Autodesk Inventor part; units mm, degrees
ref_plane "YZ Plane" through (0, 0, 0) normal (1, 0, 0) x (0, 1, 0)
ref_plane "XZ Plane" through (0, 0, 0) normal (0, 1, 0) x (-1, 0, 0)
ref_plane "XY Plane" through (0, 0, 0) normal (0, 0, 1) x (1, 0, 0)
sketch "Náčrt1" plane through (0, 0, 0) normal (0, 0, 1) x (1, 0, 0)
  line L0 (2.5, -1.4434) -> (0, -2.8868)
  line L1 (0, -2.8868) -> (-2.5, -1.4434)
  line L2 (-2.5, -1.4434) -> (-2.5, 1.4434)
  line L3 (-2.5, 1.4434) -> (0, 2.8868)
  line L4 (0, 2.8868) -> (2.5, 1.4434)
  line L5 (2.5, 1.4434) -> (2.5, -1.4434)
  circle A0 centre (0, 0) radius 1.5
  point P0 (2.5, 0)
  dimension "d1" = 3
  dimension "d16" = 5
extrude "Vysunutí1" add sketch "Náčrt1" along normal blind 20
thread "Závit1"
sketch "Náčrt2" plane through (0, 0, 20) normal (0, 0, 1) x (1, 0, 0)
  circle A0 centre (0, 0) radius 2.5
  dimension "d18" = 5
extrude "Vysunutí2" cut sketch "Náčrt2" against normal through all draft 45 keep common part
sketch "Náčrt3" plane through (0, 0, 0) normal (0, 0, -1) x (-1, 0, 0)
  circle A0 centre (0, 0) radius 2.5
  dimension "d17" = 5
extrude "Vysunutí3" cut sketch "Náčrt3" against normal through all draft 45 keep common part
chamfer "Zkosení1" distance 0.2 angle 45 1 edges at (-1.5, 0, 20)
chamfer "Zkosení2" distance 0.2 angle 45 1 edges at (-1.5, 0, 0)
properties part number "PillarBolt-M3x20" material "Ocel, vysokopevnostní, nízkolegovaná"
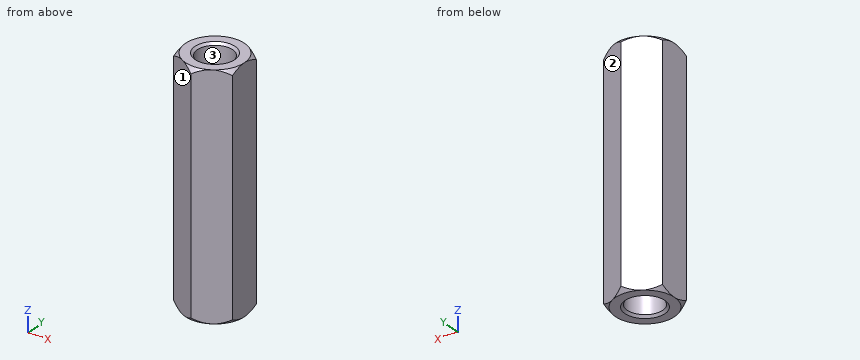
Source: CAD feature listing. Evaluate the final solid. Frame: model axes, mm. Face numbers are marked on the shaded views. Coordinates: 2 decimals unless noted, no trailing zeros. Loops run counter-clockwise (first coordinate to the right, second up) from the corner with the lowest first, then second, coordinate; pieces in that order, holes last. Notation, with made-up numbers: M -10.5,-15.5 L 15.5,-15.5 A32 cw 15.5,22.5 Z; hole C 71.25,-16 d6. An arc over 180 degrees is marked long. Put each result on its own line as item: value. Start each with the question number.
1) Contact query for flat-ended pins moving along their axis: pin 1 Ø2.5 at (x, y) = (0, 0) entering from +Z; pin 2 Ø1.5 at (y, z) = (-1.5, 17) entering from +X; pin 3 Ø1.5 at (x, z) = (2, 16) entering from -Y. Output: stop coordinate, or through.
2) Pull-direction query (Y, two-part tool) for the marked faces 1, 2 and 3; classes: pulls with the +Y half, pulls with the -Y half, needs draft (parallel to the pull), parting line crosses it, or undercut.
3) Ray query, L1, parallel to Y at x = -0.05, z = 18; L2, parallel to X at y = -0.5, z = 10; L3, parallel to Y at x = -1.25, z = 17. Return the intervals inside material, ascending. Write a range as from..to.
4) Cut plane A-A on z = 3.75. Return the cut outline in (x, y), then the cut area to 3 significant figures.
The answers:
1. pin 1: passes through
1. pin 2: stops at x = 2.5
1. pin 3: stops at y = -2.17
2. face 1: pulls with the -Y half
2. face 2: pulls with the +Y half
2. face 3: undercut
3. L1: y = -2.86..-1.5, 1.5..2.86
3. L2: x = -2.5..-1.41, 1.41..2.5
3. L3: y = -2.17..-0.83, 0.83..2.17
4. outline: M -2.5,-1.44 L 0,-2.89 L 2.5,-1.44 L 2.5,1.44 L 0,2.89 L -2.5,1.44 Z; hole C 0,0 d3
4. area: 14.6 mm²
